Can you work these out from the model? Positions are in its coordinate system, mm. Face numbers are marked on the shaded views. A direction names the side the tool comes from. Give positions to 0.01 mm unless a question says otherwise; leave off trailing zeros. Loops run counter-clockwise (first coordinate to the right, second up) from the corner with the lowest first, then second, coordinate; pieces in that order, holes last. Notation, with made-up numbers: (80.25, 3.25) - (93.25, 3.25) arc R8 ccw to (93.25, 15.25) - close; hole circle Ø11 at (79.5, 89). An arc over 180 degrees is marked (long way). Answer as a JSON object with one key per item and string values. Group by question number.
Item 1: Will these pins go through, and if not, where does the flat tip stop? pin 1 (10 mm diameter, centred on x = -29.5, y = 17.5, fed in from +Z); pin 2 (3 mm diameter, centred on x = -11, z = 1, fed in from +Y); pin 3 (3.5 mm diameter, centred on x = -8.03, z = 5, fed in from -Y).
Item 2: Suppose I cut it at B-B on y = 16. Write out the boundary of the cut face in (x, z).
Item 3: Suppose I cut it at D-D on z = 4.25. Count the separate pieces of the cut face and the enclosed holes in it, and give its area (3 significant figures).
Item 4: Thinking about a two-plate mould opening in Z: for the marked faces 4, 5 and 6, which applies, pulls with the +Z half, pulls with the -Z half, needs draft (parallel to the pull), parting line crosses it, or undercut?
Item 5: Suppose I cut it at A-A on x = -27.94. Write out the boundary of the cut face in (y, z), and give its area (3 significant figures).
Item 6: Which directions (+Z, -Z, +X, -X, +Y, -Y) give clear straight access to the entire face, cutting with the end or side of a thin tool? Please do the marked faces 1, 2 and 3.
Item 7: Suppose I cut it at C-C on x = -12.5. Write out the boundary of the cut face in (y, z).
Item 8: Please list where these lines run through material, in increasing order: L1, parallel to X at y = 25, z = 2.5; L2, parallel to Y at x = -16, z = 9.5; L3, parallel to Z at x = -27.94, y = 31.45.
from build123d import *

# Parameters (mm, degrees)
F0_W     = 35.56
F0_H     = 25.4
F1_DEPTH = 10
F3_T     = -1
F2_R     = 2.5
F2_R_2   = 1.8571721373
F2_R_3   = 1.9771948061
F2_R_4   = 1.8995875302
F4_DEPTH = 3
F5_DEPTH = 1
F6_R     = 3
F6_R_2   = 2.5
F7_DEPTH = 5
F8_DEPTH = 25.4


with BuildPart() as f1:
    # F0 (on Top) → F1 (new body)
    with BuildSketch(Plane.XY):
        with Locations((-17.78, 16.9808987513)):
            Rectangle(F0_W, F0_H)
    extrude(amount=F1_DEPTH)

    # F3
    f3_openings = [f1.faces().sort_by_distance(p)[0] for p in [
        (-17.78, 16.980899, 10),
    ]]
    offset(amount=F3_T, openings=f3_openings)

    # F2 (on face) → F4 (join)
    with BuildSketch(Plane(origin=(0, 29.6808987513, 0), x_dir=(-1, 0, 0), z_dir=(0, 1, 0))):
        with Locations((27.94, 5)):
            Circle(F2_R)
        with Locations((27.94, 5)):
            Circle(F2_R_2, mode=Mode.SUBTRACT)
        with Locations((17.94, 4.9962)):
            Circle(F2_R)
        with Locations((17.94, 4.9962)):
            Circle(F2_R_3, mode=Mode.SUBTRACT)
        with Locations((8.034, 4.9962)):
            Circle(F2_R)
        with Locations((8.034, 4.9962)):
            Circle(F2_R_4, mode=Mode.SUBTRACT)
    extrude(amount=F4_DEPTH)

    # F5 (cut, through all): faces of the model
    f5_faces = [f1.faces().sort_by_distance(p)[0] for p in [
        (-27.94, 29.6808987513, 5),
        (-17.94, 29.6808987513, 4.9962),
        (-8.034, 29.6808987513, 4.9962),
    ]]
    extrude(f5_faces, amount=-F5_DEPTH, mode=Mode.SUBTRACT)

    # F6 (on face) → F7 (join)
    with BuildSketch(Plane.XZ.offset(-4.2808987513)):
        with Locations((-17.78, 5)):
            Circle(F6_R)
        with Locations((-17.78, 5)):
            Circle(F6_R_2, mode=Mode.SUBTRACT)
    extrude(amount=F7_DEPTH)

    # F8 (cut): a face of the model
    f8_faces = [f1.faces().sort_by_distance(p)[0] for p in [
        (-17.78, 4.2808987513, 5),
    ]]
    extrude(f8_faces, amount=-F8_DEPTH, mode=Mode.SUBTRACT)


solid = f1.part
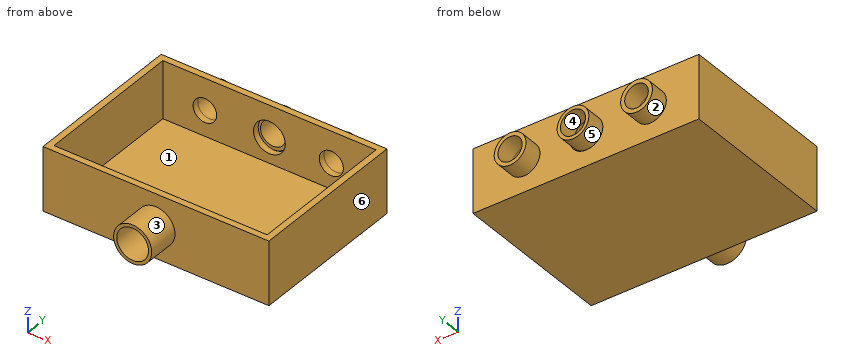
Worked out:
{
 "1": {"pin 1": "stops at z = 1", "pin 2": "stops at y = 29.68", "pin 3": "stops at y = 4.28"},
 "2": {"outline": "(-35.56, 0) - (0, 0) - (0, 10) - (-1, 10) - (-1, 1) - (-34.56, 1) - (-34.56, 10) - (-35.56, 10) - close"},
 "3": {"separate pieces": "5", "enclosed holes": "0", "area": "118 mm2"},
 "4": {"face 4": "undercut", "face 5": "parting line crosses it", "face 6": "needs draft"},
 "5": {"outline": "(4.28, 0) - (29.68, 0) - (29.68, 2.5) - (32.68, 2.5) - (32.68, 3.14) - (28.68, 3.14) - (28.68, 1) - (5.28, 1) - (5.28, 10) - (4.28, 10) - close; (28.68, 6.86) - (32.68, 6.86) - (32.68, 7.5) - (29.68, 7.5) - (29.68, 10) - (28.68, 10) - close", "area": "43.5 mm2"},
 "6": {"face 1": "+Z", "face 2": "+Y", "face 3": "-Y"},
 "7": {"outline": "(4.28, 0) - (29.68, 0) - (29.68, 10) - (28.68, 10) - (28.68, 1) - (5.28, 1) - (5.28, 10) - (4.28, 10) - close"},
 "8": {"L1": "x = -35.56 to -34.56, -1 to 0", "L2": "y = 4.28 to 5.28, 28.68 to 29.68", "L3": "z = 2.5 to 3.14, 6.86 to 7.5"}
}
